Geometry check sheet. Reference: the model listing, model coordinates, mm. A direction names the side the tool comes from. Give positions to 0.01 mm unless a question says otherwise; leave off trailing zeros. Order: outer loops, then holes, each group sorted by start corner. A loop starts at its lowest first (then second) coordinate and runs counter-clockwise, first axis right, second up. Notation, with made-up numbers: M 43.5,45 L 78.5,45 A29 cw 78.5,83 Z; hole C -32,-38.75 d1. An arc over 180 degrees is marked long. Answer as CSV lines item,"result".
Autodesk Inventor part; units mm, degrees
ref_plane "YZ Plane" through (0, 0, 0) normal (1, 0, 0) x (0, 1, 0)
ref_plane "XZ Plane" through (0, 0, 0) normal (0, 1, 0) x (-1, 0, 0)
ref_plane "XY Plane" through (0, 0, 0) normal (0, 0, 1) x (1, 0, 0)
sketch "Sketch1" plane through (0, 0, 0) normal (0, 0, 1) x (1, 0, 0)
  line L0 (-50, -150) -> (50, -150)
  line L1 (50, -150) -> (50, 150)
  line L2 (50, 150) -> (-50, 150)
  line L3 (-50, 150) -> (-50, -150)
  line L4 (-50, -150) -> (50, 150) construction
  line L5 (50, -150) -> (-50, 150) construction
  point P0 (0, 0)
  dimension "d0" = 100
  dimension "d1" = 300
extrude "Extrusion1" add sketch "Sketch1" along normal blind 5
sketch "Sketch2" plane through (-50, 150, 0) normal (0, 1, 0) x (1, 0, 0)
  line L0 (0, 0) -> (100, 0)
  line L1 (0, 0) -> (49.9986, 49.9986)
  line L2 (49.9986, 49.9986) -> (53.5341, 46.463)
  line L3 (53.5341, 46.463) -> (3.5355, -3.5355)
  line L4 (3.5355, -3.5355) -> (0, 0)
  line L5 (0, 0) -> (70.7086, 0) construction
  line L6 (100.108, -0.1109) -> (53.5341, 46.463)
  line L7 (53.5341, 46.463) -> (49.9986, 42.9275)
  line L8 (49.9986, 42.9275) -> (96.5724, -3.6464)
  line L9 (96.5724, -3.6464) -> (100.108, -0.1109)
  point P0 (50, 0)
  point P1 (49.9986, 42.9275)
  dimension "d4" = 45
  dimension "d5" = 5
  dimension "d6" = 5
extrude "Extrusion2" add sketch "Sketch2" against normal blind 150 contours L1 L2 L3 L0 | L0 L3 L4 | L8 L3 L6 L0 | L0 L6 L9 L8
sketch "Sketch7" plane through (0, 0, 5) normal (0, 0, 1) x (1, 0, 0)
  line L0 (4.9986, 125) -> (-5.0014, 125)
  line L1 (-25.0014, 105) -> (-25.0014, 95)
  line L2 (-5.0014, 75) -> (4.9986, 75)
  line L3 (24.9986, 95) -> (24.9986, 105)
  line L4 (-0.0014, 150) -> (-0.0014, 0)
  line L5 (24.9986, 125) -> (-25.0014, 75) construction
  line L6 (-25.0014, 125) -> (24.9986, 75) construction
  arc A0 (4.9986, 75) -> (24.9986, 95) centre (4.9986, 95) ccw
  arc A1 (24.9986, 105) -> (4.9986, 125) centre (4.9986, 105) ccw
  arc A2 (-5.0014, 125) -> (-25.0014, 105) centre (-5.0014, 105) ccw
  arc A3 (-25.0014, 95) -> (-5.0014, 75) centre (-5.0014, 95) ccw
  point P0 (0, 0)
  point P1 (-0.0014, 100)
  dimension "d26" = 50
  dimension "d27" = 50
  dimension "d28" = 20
extrude "Extrusion7" cut sketch "Sketch7" against normal blind 5
properties part number "fixation_v06"
(1) Gauge pin test, flat ends, axial feed: P1, Ø8, axis at x = 8, y = 77, coming from the -Z side; P2, Ø8, axis at y = 71, z = -25.5, coming from the -X side; P3, Ø2, axis at x = 32.5, z = -21, coming from the +Y side; P4, Ø1.5, axis at y = 101.5, z = 2.5, coming from the +X side. Record the tip position at first contact, or that the pin passes through.
The answers:
P1,"stops at z = -46"
P2,"stops at x = -28.5"
P3,"passes through"
P4,"stops at x = 50"
(2) Section check B-B on x = 13. Enter the section's corners in (y, z).
The answers:
outline,"M -150,0 L 76.67,0 L 76.67,5 L -150,5 Z; M 0,-37 L 150,-37 L 150,-29.93 L 0,-29.93 Z; M 123.33,0 L 150,0 L 150,5 L 123.33,5 Z"
(3) Material ranges on line 1 (X direction, y = 90, z = -45); line 2 (X direction, y = 55, z = -29); line 3 (Z direction, x = -12.5, y = 53), recorded low to high.
The answers:
line 1,"x = -5 to 5"
line 2,"x = -21 to -13.93, 13.93 to 21"
line 3,"z = -37.5 to -30.43, 0 to 5"
(4) Tool access check on faces 5 (the face through (-1, 2, 5)), 6 (the face through (-21.165, 76.05, -21.764)), 7 (the face through (-19.298, 81.014, 2.535)). Record the directions out of +Z, -Z, +X, -X, +Y, -Y that give a thin tool (end or side, any length) a straight path to the whole face; none if there is none.
The answers:
face 5,"+Z, +X, -X, +Y, -Y"
face 6,"+Y, -Y"
face 7,"+Z"
(5) Section check C-C on x = -33.5. Enter the section's corners in (y, z).
The answers:
outline,"M -150,0 L 150,0 L 150,5 L -150,5 Z; M 0,-16.5 L 150,-16.5 L 150,-9.43 L 0,-9.43 Z"
(6) Draft check along X on faces 1 (the face through (24.999, 100, 3)), 2 (the face through (50, -2, 2)), 3 (the face through (-11, 0, -33)), 4 (the face through (21.162, 76.05, -21.764)). Enter one of: +X half, -X half, draft (parallel to the pull), parting line (faces both ways), or undercut.
The answers:
face 1,"undercut"
face 2,"+X half"
face 3,"draft"
face 4,"undercut"
(7) Section check D-D on z = -30. Enter the section's corners in (x, y), then the cut area to 3 significant figures.
The answers:
outline,"M -20,0 L -12.93,0 L -12.93,150 L -20,150 Z; M 12.93,0 L 20,0 L 20,150 L 12.93,150 Z"
area,"2,120 mm2"
